from build123d import *

# Parameters (mm, degrees)
F1_DEPTH = 3


with BuildPart() as f1:
    # F0 (on Top) → F1 (new body)
    with BuildSketch(Plane.XY):
        with BuildLine():
            Line((-3, 0), (-1, 0))
            ThreePointArc((-1, 0), (-0.292893, 0.292893), (0, 1))
            Line((0, 1), (0, 5))
            ThreePointArc((0, 5), (-0.292893, 5.707107), (-1, 6))
            Line((-1, 6), (-9, 6))
            ThreePointArc((-9, 6), (-9.707107, 5.707107), (-10, 5))
            Line((-10, 5), (-10, 1))
            ThreePointArc((-10, 1), (-9.707107, 0.292893), (-9, 0))
            Line((-9, 0), (-7, 0))
            ThreePointArc((-7, 0), (-6.292893, -0.292893), (-6, -1))
            Line((-6, -1), (-6, -6.5))
            ThreePointArc((-6, -6.5), (-5.707107, -7.207107), (-5, -7.5))
            Line((-5, -7.5), (-3, -7.5))
            ThreePointArc((-3, -7.5), (-2.292893, -7.207107), (-2, -6.5))
            Line((-2, -6.5), (-2, -5.5))
            ThreePointArc((-2, -5.5), (-2.292893, -4.792893), (-3, -4.5))
            Line((-3, -4.5), (-4, -4.5))
            Line((-4, -4.5), (-4, -1))
            ThreePointArc((-4, -1), (-3.707107, -0.292893), (-3, 0))
        make_face()
    extrude(amount=F1_DEPTH)


solid = f1.part
Can you work these out from the model? Positions are in its coordinate system, mm. A direction names the side the tool comes from. Give positions to 0.01 mm unless a question says otherwise; leave off trailing zeros. Loops run counter-clockwise (first coordinate to the right, second up) from the corner with the lowest first, then second, coordinate; pieces in that order, holes last. Notation, with made-up numbers: (12.25, 58.5) - (47.25, 58.5) arc R29 ccw to (47.25, 79.5) - close; hole circle Ø3 at (-11.75, -4.75). An arc over 180 degrees is marked (long way). One line per item, written item: value.
(1) If we section it at A-A, the plane x = -3.5: List the corners of the cut face in (y, z) for me, plus the area to 3 significant figures.
Verdict:
outline: (-7.5, 0) - (-4.5, 0) - (-4.5, 3) - (-7.5, 3) - close; (-0.13, 0) - (6, 0) - (6, 3) - (-0.13, 3) - close
area: 27.4 mm^2
(2) On a 3-axis mill with a long thin cutter (end or side, diameter ignored), from which of +Z, -Z, +X, -X, +Y, -Y can I reach the whole of each face in a straight line? I mean faces 1 (the face through (-8, 0, 1)), 2 (the face through (-5, 1, 0)), 3 (the face through (-2, -6, 1)), 4 (the face through (-2.285, -4.801, 1.479)). Say none if no direction works.
Verdict:
face 1: +Z, -Z, -X, -Y
face 2: -Z, +X, -X, +Y, -Y
face 3: +Z, -Z, +X, -Y
face 4: +Z, -Z, +X
(3) If we mould it in two halves opening along Y, with no side actions, what happens to faces 5 (the face through (-0.285, 5.699, 1.479)), 6 (the face through (-3.5, -4.5, 1.5)), 7 (the face through (-9.715, 0.301, 1.479))? For each: released by +Y, released by -Y, zero draft, split by the parting line, or undercut.
Verdict:
face 5: released by +Y
face 6: undercut
face 7: released by -Y
(4) I need wall thicknesses on line 1 along Y through (x, z) = (-1.5, 1.15); line 2 along X through (y, z) = (-6.5, 1.95); line 3 along X through (y, z) = (-4, 2.5). Which ranges of each line are inside material? Lowest first, please.
Verdict:
line 1: 0 to 6
line 2: -6 to -2
line 3: -6 to -4
(5) If we section it at B-B, the plane z = 1.9: List the corners of the cut face in (x, y) for me.
Verdict:
outline: (-10, 1) arc R1 ccw to (-9, 0) - (-7, 0) arc R1 cw to (-6, -1) - (-6, -6.5) arc R1 ccw to (-5, -7.5) - (-3, -7.5) arc R1 ccw to (-2, -6.5) - (-2, -5.5) arc R1 ccw to (-3, -4.5) - (-4, -4.5) - (-4, -1) arc R1 cw to (-3, 0) - (-1, 0) arc R1 ccw to (0, 1) - (0, 5) arc R1 ccw to (-1, 6) - (-9, 6) arc R1 ccw to (-10, 5) - close
(6) I'm going to push flat-ended pins straight in: pin 1 (0.6 mm diameter, centred on x = -8, z = 1.5, fed in from -Y); pin 2 (1.5 mm diameter, centred on y = -3.5, z = 2, fed in from -X); pin 3 (1.6 mm diameter, centred on x = -2, z = 2, fed in from -Y). Where does each tip first touch, or does it pass through?
Verdict:
pin 1: y = 0
pin 2: x = -6
pin 3: y = -7.48
(7) If we section it at D-D, the plane x = -1.75: List the corners of the cut face in (y, z) for me.
Verdict:
outline: (0, 0) - (6, 0) - (6, 3) - (0, 3) - close
(8) If we section it at C-C, the plane y = -2.25: List the corners of the cut face in (x, z) for me.
Verdict:
outline: (-6, 0) - (-4, 0) - (-4, 3) - (-6, 3) - close
